Could you check a few things on this drawing? It's one solid part, dimensions in mm from its lowest x, y, z. A direction names the side the tool comes from. Coordinates: 2 decimals unless noted, no trailing zeros. Order: outer loops, then holes, each group sorted by start corner. A loop starts at its lowest first (then second) coordinate and runs counter-clockwise, first axis right, second up.
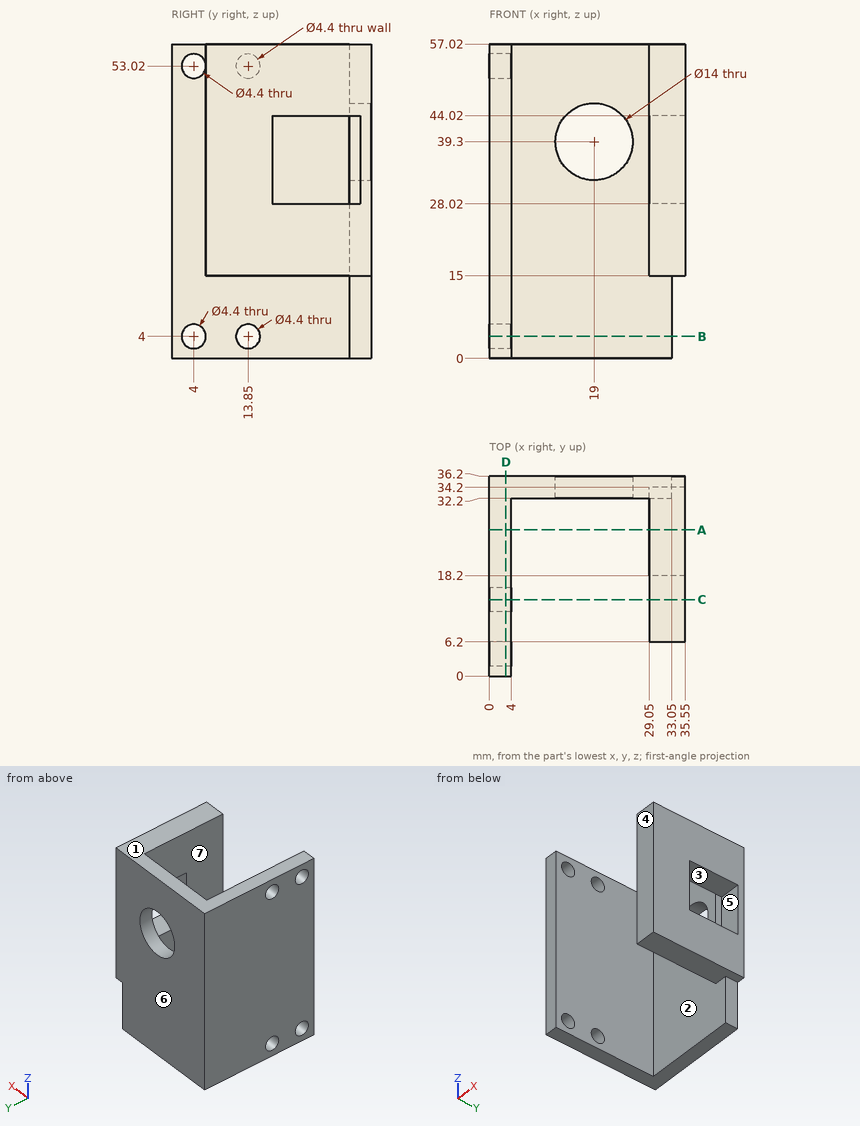
Q1. If we section it at D-D on x = 3: Write out the boundary of the cut face in (y, z).
Q2. I need wall thicknesses on L1, parallel to Y at x = 1.5, z = 4; L2, parallel to X at y = 15, z = 29; L3, parallel to Y at x = 2, z = 52. Which ranges of each line are inside material? Lowest first, please.
Q3. We'd pull the mould along Z, two halves only. Please class the marked faces 1, 2 and 3: pulls with the +Z half, pulls with the -Z half, needs draft (parallel to the pull), parting line crosses it, or undercut.
Q4. If we section it at A-A on y = 26.5: Write out the boundary of the cut face in (x, z).
Q5. If we section it at C-C on y = 13.85: Write out the boundary of the cut face in (x, z), then the cut area to 3 significant figures.
Q6. For the marked faces 4, 5, 6 and 7, which set-ups out of +Z, -Z, +X, -X, +Y, -Y let a thin tool reach every point of the face, with its end or its side?
Q7. If we section it at B-B on z = 4: Write out the boundary of the cut face in (x, y).
Q8. Will these pins go through, and if not, where does the flat tip stop? pin 1 (1 mm diameter, centred on x = 30.5, y = 26.5, fed in from -Z); pin 2 (1.2 mm diameter, centred on y = 34, z = 9, fed in from +X); pin 3 (3 mm diameter, centred on x = 34, z = 35, fed in from -Y).
Reply:
1. outline: (0, 0) - (36.2, 0) - (36.2, 57.02) - (0, 57.02) - close; hole circle Ø4.4 at (4, 4); hole circle Ø4.4 at (4, 53.02); hole circle Ø4.4 at (13.85, 4); hole circle Ø4.4 at (13.85, 53.02)
2. L1: y = 0 to 1.8, 6.2 to 11.65, 16.05 to 36.2
2. L2: x = 0 to 4, 29.05 to 35.55
2. L3: y = 0 to 2.05, 5.95 to 11.9, 15.8 to 36.2
3. face 1: pulls with the +Z half
3. face 2: needs draft
3. face 3: undercut
4. outline: (0, 0) - (4, 0) - (4, 57.02) - (0, 57.02) - close; (29.05, 15) - (35.55, 15) - (35.55, 28.02) - (29.05, 28.02) - close; (29.05, 44.02) - (35.55, 44.02) - (35.55, 57.02) - (29.05, 57.02) - close
5. outline: (0, 0) - (4, 0) - (4, 1.8) - (0, 1.8) - close; (0, 6.2) - (4, 6.2) - (4, 50.82) - (0, 50.82) - close; (0, 55.22) - (4, 55.22) - (4, 57.02) - (0, 57.02) - close; (29.05, 15) - (35.55, 15) - (35.55, 57.02) - (29.05, 57.02) - close
5. area: 466 mm2
6. face 4: +Z, -Z, +X, -Y
6. face 5: +X
6. face 6: +Z, -Z, +X, -X, +Y
6. face 7: +Z, -Z, -Y
7. outline: (0, 0) - (4, 0) - (4, 1.8) - (0, 1.8) - close; (0, 6.2) - (4, 6.2) - (4, 11.65) - (0, 11.65) - close; (0, 16.05) - (4, 16.05) - (4, 32.2) - (33.05, 32.2) - (33.05, 36.2) - (0, 36.2) - close
8. pin 1: stops at z = 15
8. pin 2: stops at x = 33.05
8. pin 3: stops at y = 6.2
